Drawing for the job (mm, zero at the part's lowest x, y, z). A direction names the side the tool comes from. Give positions to 0.01 mm unless a question says otherwise; leave off trailing zeros. Loops run counter-clockwise (first coordinate to the right, second up) from the corner with the lowest first, then second, coordinate; pieces in that order, holes last. Notation, with made-up numbers: (8, 60.5) -> (45, 60.5) arc R19 cw to (45, 95.5) -> close; hole circle Ø1 at (31, 40.5). An arc over 180 degrees is marked (long way). Use CSV: the item, a comma, the result in double quotes. Start each with the question number.
(1) Drill centre lines: probe 1 along X at (y, z) = (9.5, 17.5); probe 2 along X at (y, z) = (6.75, 48); probe 3 along Z at (x, y) = (31, 2.75). Where is each one in solid material? Low to high.
(2) Pull direction X, two halves, no side cores. Call the marked faces 1 and 2: pulls with the +X half, pulls with the -X half, needs draft (parallel to the pull), parting line crosses it, or undercut.
(3) 3-axis set-ups, long thin cutter, end or side, ignore diameter. For the marked faces 3 and 4: which of +Z, -Z, +X, -X, +Y, -Y reach the whole face in a straight line?
(4) Cut at A-A on z = 31. Write the cut outline in (x, y).
(5) Cut at D-D on y = 6.5. Write the cut outline in (x, z), then the cut area to 3 significant figures.
(6) Cut at B-B on y = 3. Write the cut outline in (x, z), then the cut area to 3 significant figures.
(7) Cut at C-C on x = 39. Write the cut outline in (y, z).
(8) Flat gauge pins, fed straight in: pin 1 (5.5 mm diameter, centred on y = 3.5, z = 61, fed in from +X); pin 2 (1.5 mm diameter, centred on y = 3.5, z = 54, fed in from +X); pin 3 (4 mm diameter, centred on x = 16, y = 6.5, fed in from +Z); pin 4 (12 mm diameter, centred on x = 57, z = 18, fed in from -Y). Where does each tip first touch, or does it go through?
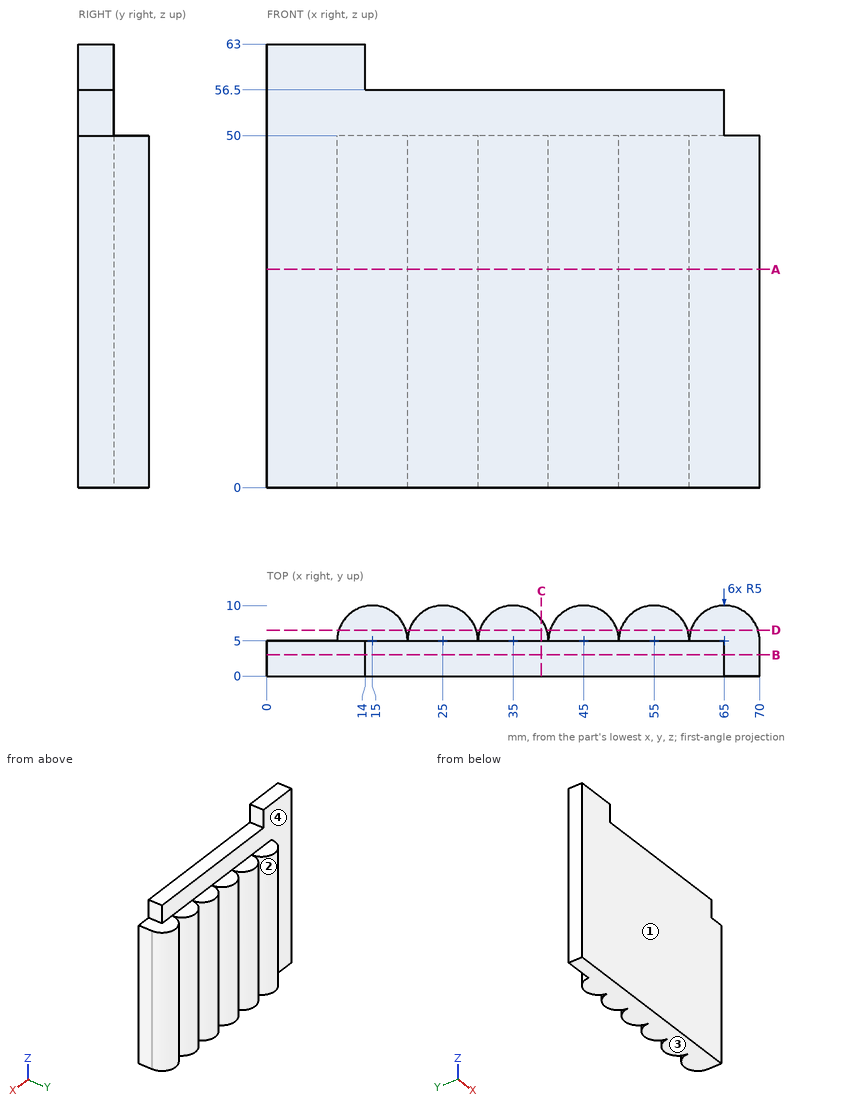
Check result:
1,probe 1,"12.82 to 17.18, 22.82 to 27.18, 32.82 to 37.18, 42.82 to 47.18, 52.82 to 57.18, 62.82 to 67.18"
1,probe 2,"10.32 to 19.68, 20.32 to 29.68, 30.32 to 39.68, 40.32 to 49.68, 50.32 to 59.68, 60.32 to 69.68"
1,probe 3,"0 to 56.5"
2,face 1,"needs draft"
2,face 2,"undercut"
3,face 3,"-Z, +X, -X, +Y, -Y"
3,face 4,"+Z, -X, +Y"
4,outline,"(0, 0) -> (70, 0) -> (70, 5) arc R5 ccw to (60, 5) arc R5 ccw to (50, 5) arc R5 ccw to (40, 5) arc R5 ccw to (30, 5) arc R5 ccw to (20, 5) arc R5 ccw to (10, 5) -> (0, 5) -> close"
5,outline,"(10.23, 0) -> (19.77, 0) -> (19.77, 50) -> (10.23, 50) -> close; (20.23, 0) -> (29.77, 0) -> (29.77, 50) -> (20.23, 50) -> close; (30.23, 0) -> (39.77, 0) -> (39.77, 50) -> (30.23, 50) -> close; (40.23, 0) -> (49.77, 0) -> (49.77, 50) -> (40.23, 50) -> close; (50.23, 0) -> (59.77, 0) -> (59.77, 50) -> (50.23, 50) -> close; (60.23, 0) -> (69.77, 0) -> (69.77, 50) -> (60.23, 50) -> close"
5,area,"2,860 mm²"
6,outline,"(0, 0) -> (70, 0) -> (70, 50) -> (65, 50) -> (65, 56.5) -> (14, 56.5) -> (14, 63) -> (0, 63) -> close"
6,area,"4,010 mm²"
7,outline,"(0, 0) -> (8, 0) -> (8, 50) -> (5, 50) -> (5, 56.5) -> (0, 56.5) -> close"
8,pin 1,"x = 14"
8,pin 2,"x = 65"
8,pin 3,"z = 56.5"
8,pin 4,"y = 0"
